from build123d import *

# Parameters (mm, degrees)
F0_W     = 127
F0_H     = 76.2
F0_R     = 19.05
F1_DEPTH = 25.4
F2_R     = 12.7
F3_DEPTH = 25.4
F5_DEPTH = 128.778


with BuildPart() as f1:
    # F0 (on Top) → F1 (new body)
    with BuildSketch(Plane.XY):
        Rectangle(F0_W, F0_H)
        Circle(F0_R, mode=Mode.SUBTRACT)
        Circle(F0_R)
    extrude(amount=F1_DEPTH)

    # F2 (on face) → F3 (cut)
    with BuildSketch(Plane.XY.offset(25.4)):
        Circle(F2_R)
    extrude(amount=-F3_DEPTH, mode=Mode.SUBTRACT)

    # F4 (on face) → F5 (cut)
    with BuildSketch(Plane.YZ.offset(63.5)):
        Polygon((38.1, 0), (38.1, 5.679613), (33.02, 0), align=None)
    extrude(amount=-F5_DEPTH, mode=Mode.SUBTRACT)


solid = f1.part
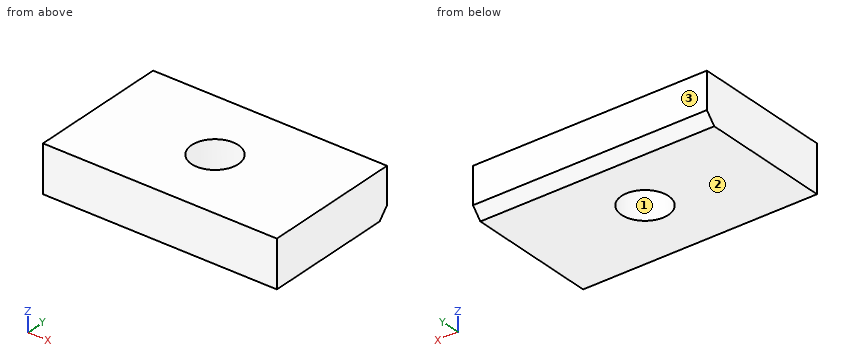
Can you work these out from the model? Positions are in its coordinate system, mm. Face numbers are marked on the shaded views. Give positions to 0.01 mm unless a question says otherwise; leave off trailing zeros. Loops run counter-clockwise (first coordinate to the right, second up) from the corner with the lowest first, then second, coordinate; pieces in that order, holes last. Notation, with made-up numbers: (77.25, 89) -> (123.25, 89) arc R12 ccw to (123.25, 108) -> close; hole circle Ø3 at (-20, 11.5). An arc over 180 degrees is marked (long way). Use one line per item in the form item = value.
1) We'd pull the mould along Y, two halves only. Please class the marked faces 1, 2 and 3: released by +Y, released by -Y, zero draft, split by the parting line, or undercut.
Answers:
face_1 = undercut
face_2 = zero draft
face_3 = released by +Y
2) If we section it at B-B (y = 0): Please give me the cut outline in (x, z), plus the area to 3 significant figures.
Answers:
outline = (-63.5, 0) -> (-12.7, 0) -> (-12.7, 25.4) -> (-63.5, 25.4) -> close; (12.7, 0) -> (63.5, 0) -> (63.5, 25.4) -> (12.7, 25.4) -> close
area = 2,580 mm²
3) I need wall thicknesses on line 1 along Y through (x, z) = (0, 10.5); line 2 along X through (y, z) = (7, 18.5); line 3 along Y through (x, z) = (-2.5, 22.75). Which ranges of each line are inside material? Lowest first, please.
Answers:
line_1 = -38.1 to -12.7, 12.7 to 38.1
line_2 = -63.5 to -10.6, 10.6 to 63.5
line_3 = -38.1 to -12.45, 12.45 to 38.1
4) If we section it at C-C (z = 13): Please give me the cut outline in (x, y), plus the area to 3 significant figures.
Answers:
outline = (-63.5, -38.1) -> (63.5, -38.1) -> (63.5, 38.1) -> (-63.5, 38.1) -> close; hole circle Ø25.4 at (0, 0)
area = 9,170 mm²
5) If we section it at A-A (x = 0): Please give me the cut outline in (y, z).
Answers:
outline = (-38.1, 0) -> (-12.7, 0) -> (-12.7, 25.4) -> (-38.1, 25.4) -> close; (12.7, 0) -> (33.02, 0) -> (38.1, 5.68) -> (38.1, 25.4) -> (12.7, 25.4) -> close
6) If we section it at D-D (y = 8.5): Please give me the cut outline in (x, z), plus the area to 3 significant figures.
Answers:
outline = (-63.5, 0) -> (-9.44, 0) -> (-9.44, 25.4) -> (-63.5, 25.4) -> close; (9.44, 0) -> (63.5, 0) -> (63.5, 25.4) -> (9.44, 25.4) -> close
area = 2,750 mm²
